CAD build for the part. Positions are in the model's coordinates, mm. Give positions to 0.01 mm unless a question says otherwise; leave off trailing zeros. Order: outer loops, then holes, each group sorted by start corner. A loop starts at its lowest first (then second) coordinate and runs counter-clockwise, first axis right, second up. Notation, with made-up numbers: (48, 50) -> (87, 50) arc R21 ccw to (87, 79) -> close; hole circle Ø6 at (-30, 19.25). An arc over 180 degrees is marked (long way). Use one line per item in the form item = value. Start each with the question number.
1) Cut at C-C, the plane y = -9.5. Give the cut face in (x, z), and give its area (3 significant figures).
2) Cut at B-B, the plane x = 0. Give the cut face in (y, z).
3) Drop a flat-ended pin along its axis: P1, Ø4, axis at x = -2, z = 2, coming from the +Y side. Give the stop position or say it passes through.
4) Cut at A-A, the plane z = 0. Give the cut face in (x, y).
5) Probe line 1 (Z direction, x = 0, y = -12); line 2 (X direction, y = -27.5, z = 0.5); line 3 (Y direction, x = -2.5, z = -1.75). List the from-to ranges inside material, lowest first.
from build123d import *

# Parameters (mm, degrees)
F0_R        = 2.5
F1_DEPTH    = 25
F2_R        = 3.5
F2_R_2      = 2.5
F3_DEPTH    = 7
F4_S5_R     = 2.5
F4_T6_DEPTH = 7


# Not quite as in the source:
# - a fillet or chamfer that OpenCascade refuses, or shapes differently, is made with other operations: its cross-section is extruded or revolved along the edge and cut away or added


with BuildPart() as f1:
    # F0 (on Front) → F1 (new body)
    with BuildSketch(Plane.XZ):
        Circle(F0_R)
    extrude(amount=F1_DEPTH)

    # F2 (on face) → F3 (join)
    with BuildSketch(Plane.XZ.offset(25)):
        Circle(F2_R)
        Circle(F2_R_2, mode=Mode.SUBTRACT)
        Circle(F2_R_2)
    extrude(amount=F3_DEPTH)

    # F4: chamfer of 2 on 1 edges, made by hand


with BuildPart() as f4_tool2:
    # F4_s3 → F4_t4 (revolve)
    with BuildSketch(Plane.XY):
        Polygon((3.5, -27), (1.5, -25), (3.5, -25), align=None)
    revolve(axis=Axis((0, -25, 0), (0, -1, 0)))

    # F4_s5 → F4_t6 (cut, symmetric)
    with BuildSketch(Plane.XZ.offset(26)):
        Circle(F4_S5_R)
    extrude(amount=F4_T6_DEPTH, both=True, mode=Mode.SUBTRACT)


with BuildPart() as f1_1:
    add(f1.part)

    # F4_t1: cut F4_tool2
    add(f4_tool2.part, mode=Mode.SUBTRACT)


solid = f1_1.part
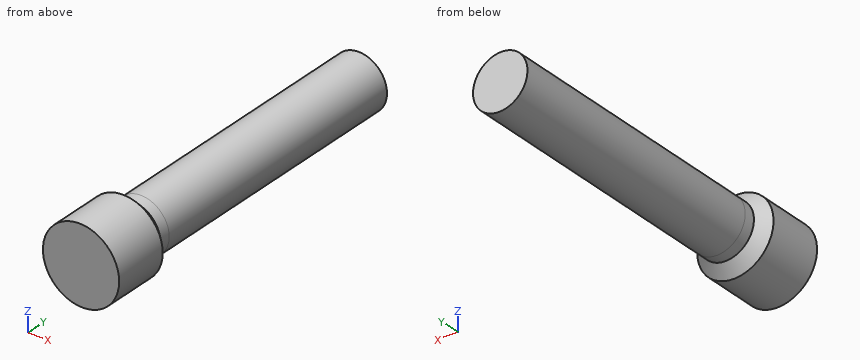
Result:
q1.outline = circle Ø5 at (0, 0)
q1.area = 19.6 mm²
q2.outline = (-32, -3.5) -> (-27, -3.5) -> (-26, -2.5) -> (0, -2.5) -> (0, 2.5) -> (-26, 2.5) -> (-27, 3.5) -> (-32, 3.5) -> close
q3.P1 = 0
q4.outline = (-3.5, -32) -> (3.5, -32) -> (3.5, -27) -> (2.5, -26) -> (2.5, 0) -> (-2.5, 0) -> (-2.5, -26) -> (-3.5, -27) -> close
q5.line_1 = -2.5 to 2.5
q5.line_2 = -3.46 to 3.46
q5.line_3 = -32 to -26.55
